Check sheet for the modelled part. Datum: model origin and axes. Units: mm. A direction names the side the tool comes from. Round coordinates to 2 decimals unless told otherwise and drop trailing zeros. Write each loop counter-clockwise with the first axis right and the second up, starting at its lowest first coordinate (ties: lowest second). Pieces come first, ordered by that corner, then holes. Notation, with made-up numbers: M 69.5,34.25 L 88.5,34.25 A22 cw 88.5,46.25 Z; hole C -26.75,-16 d4. An arc over 180 degrees is marked long. Put each result on its own line as item: value.
```python
from build123d import *

# Parameters (mm, degrees)
F0_R     = 19
F1_DEPTH = 57.1
F2_R     = 16
F3_DEPTH = 28.5
F4_R     = 10
F5_DEPTH = 3
F6_R     = 3
F7_DEPTH = 16.2
F9_D     = 3
F9_DEPTH = 5
F9_TIP   = 0.9012909285


with BuildPart() as f1:
    # F0 (on Top) → F1 (new body)
    with BuildSketch(Plane.XY):
        Circle(F0_R)
    extrude(amount=F1_DEPTH)

    # F2 (on face) → F3 (join)
    with BuildSketch(Plane.XY.offset(57.1)):
        Circle(F2_R)
    extrude(amount=F3_DEPTH)

    # F4 (on face) → F5 (join)
    with BuildSketch(Plane.XY.offset(85.6)):
        Circle(F4_R)
    extrude(amount=F5_DEPTH)

    # F6 (on face) → F7 (join)
    with BuildSketch(Plane.XY.offset(88.6)):
        Circle(F6_R)
    extrude(amount=F7_DEPTH)

    # F9
    with Locations(Plane.XY.offset(85.6)):
        with Locations((-9.1923881554, 9.1923881554), (9.1923881554, 9.1923881554), (9.1923881554, -9.1923881554), (-9.1923881554, -9.1923881554)):
            Hole(F9_D / 2, depth=F9_DEPTH)
            with Locations((0, 0, -(F9_DEPTH + F9_TIP / 2))):  # 118° drill point
                Cone(0, F9_D / 2, F9_TIP, mode=Mode.SUBTRACT)


solid = f1.part
```
1. Cross-section at D-D (x = 13). Enter the section's corners in (y, z), then the cut area to 3 significant figures.
Computed values:
outline: M -13.86,0 L 13.86,0 L 13.86,57.1 L 9.33,57.1 L 9.33,85.6 L -9.33,85.6 L -9.33,57.1 L -13.86,57.1 Z
area: 2,110 mm2
2. Cross-section at A-A (y = 0). Enter the section's corners in (x, z), then the cut area to 3 significant figures.
Computed values:
outline: M -19,0 L 19,0 L 19,57.1 L 16,57.1 L 16,85.6 L 10,85.6 L 10,88.6 L 3,88.6 L 3,104.8 L -3,104.8 L -3,88.6 L -10,88.6 L -10,85.6 L -16,85.6 L -16,57.1 L -19,57.1 Z
area: 3,240 mm2
3. Scan lines: probe 1 along Z at (x, y) = (0.5, 6.5); probe 2 along Y at (x, z) = (9.5, 82.5); probe 3 along Z at (x, y) = (3, -11). Record each from-to range of solid material in increasing order.
Computed values:
probe 1: z = 0 to 88.6
probe 2: y = -12.87 to -10.66, -7.72 to 7.72, 10.66 to 12.87
probe 3: z = 0 to 85.6
4. Access from +Z, -Z, +X, -X, +Y, -Y to the whole of each face (thin tool, end or side, straight path). Record for faces 1 (the flat face through (2.1, 2.4, 88.6)), 2 (the cylindrical face through (8.767, -16.856, 28.15)).
Computed values:
face 1: +Z
face 2: +Z, -Z
5. Cross-section at C-C (z = 30). Enter the section's corners in (x, y).
Computed values:
outline: C 0,0 d38
6. Depth check by flat-ended pin: pin 1 Ø8 at (x, z) = (15, 42.5) entering from +Y; pin 2 Ø2 at (x, z) = (-7.5, 44) entering from +Y; pin 3 Ø12 at (x, y) = (-13, -3) entering from +Z. Enter the tip coordinate at first touch or a pass-through.
Computed values:
pin 1: stops at y = 15.49
pin 2: stops at y = 17.85
pin 3: stops at z = 88.6
7. Release check for a two-part mould opening along X. For faces 3 (the cylindrical face through (-3, 0, 97)), 4 (the flat face through (0, 0, 104.8)), 5 (the cylindrical face through (9.52, 7.73, 83.06)) record: +X half, -X half, draft (parallel to the pull), parting line (faces both ways), or undercut.
Computed values:
face 3: parting line
face 4: draft
face 5: undercut
